```python
from build123d import *

# Parameters (mm, degrees)
F0_W     = 30
F0_H     = 100
F1_DEPTH = 10
F2_W     = 17
F2_H     = 10
F3_DEPTH = 200
F2_H_2   = 5
F4_DEPTH = 60
F5_R     = 1.25
F6_DEPTH = 25
F7_R     = 1.25
F8_DEPTH = 25


with BuildPart() as f1:
    # F0 (on Top) → F1 (new body, symmetric)
    with BuildSketch(Plane.XY):
        Rectangle(F0_W, F0_H)
    extrude(amount=F1_DEPTH, both=True)

    # F2 (on face) → F3 (cut)
    with BuildSketch(Plane.XZ.offset(50)):
        Rectangle(F2_W, F2_H)
    extrude(amount=-F3_DEPTH, mode=Mode.SUBTRACT)

    # F2 (on face) → F4 (cut)
    with BuildSketch(Plane.XZ.offset(50)):
        Polygon((8.5, 10), (8.5, 5), (8.5, -5), (10.5, -5), (10.5, 10), align=None)
        Polygon((-8.5, -5), (-8.5, 5), (-8.5, 10), (-10.5, 10), (-10.5, -5), align=None)
        with Locations((0, 7.5)):
            Rectangle(F2_W, F2_H_2)
    extrude(amount=-F4_DEPTH, mode=Mode.SUBTRACT)

    # F5 (on face) → F6 (cut)
    with BuildSketch(Plane.XY.offset(-5)):
        with Locations((0, -18.688429)):
            Circle(F5_R)
        with Locations((0, -40.465806)):
            Circle(F5_R)
    extrude(amount=-F6_DEPTH, mode=Mode.SUBTRACT)

    # F7 (on face) → F8 (cut)
    with BuildSketch(Plane.XY.offset(10)):
        with Locations((0, 30.281067)):
            Circle(F7_R)
    extrude(amount=-F8_DEPTH, mode=Mode.SUBTRACT)


solid = f1.part
```
Source: CAD feature listing. Evaluate the final solid. Frame: model axes, mm. A direction names the side the tool comes from. Round coordinates to 2 decimals unless told otherwise and drop trailing zeros. Loops run counter-clockwise (first coordinate to the right, second up) from the corner with the lowest first, then second, coordinate; pieces in that order, holes last.
1. Section query D-D on y = 36. Output: boundary loops of the cut face in (x, z).
2. Access query for faces 4 (the flat face through (0, -1, -5)), 5 (the flat face through (-10.5, -20, 3)), 6 (the flat face through (8.5, 30, 0)). Directions: +Z, -Z, +X, -X, +Y, -Y. A direction counts if a zero-diameter tool reaches every point of the face in a straight line with its end or side. Return the directions, or none.
3. Ray query, L1, parallel to Y at x = 0, z = -6.4; L2, parallel to X at y = 8, z = 5; L3, parallel to Z at x = -3, y = 28. Return the intervals inside material, ascending.
4. Section query C-C on x = -5.25. Output: boundary loops of the cut face in (y, z).
5. Section query B-B on z = -3. Output: boundary loops of the cut face in (x, y).
6. Mould query, pull axis Y, two halves, no side actions, for faces 1 (the flat face through (-15, -1, 0)), 2 (the cylindrical face through (-0.271, -41.686, -7.465)), 3 (the flat face through (0, 50, 7)). Classes: released by +Y, released by -Y, zero draft, split by the parting line, or undercut.
7. Section query A-A on x = 0. Output: boundary loops of the cut face in (y, z).
8. Contact query for flat-ended pins moving along their axis: pin 1 (12 mm diameter, centred on x = -1.5, z = 5.5, fed in from -Y); pin 2 (2 mm diameter, centred on x = 0, y = 30.28, fed in from +Z). Output: stop coordinate, or through.
Answers below:
1. outline: (-15, -10) - (15, -10) - (15, 10) - (-15, 10) - close; hole (-8.5, -5) - (8.5, -5) - (8.5, 5) - (-8.5, 5) - close
2. face 4: -Y
2. face 5: +Z, -Y
2. face 6: +Y, -Y
3. L1: y = -50 to -41.72, -39.22 to -19.94, -17.44 to 29.03, 31.53 to 50
3. L2: x = -15 to -10.5, 10.5 to 15
3. L3: z = -10 to -5, 5 to 10
4. outline: (-50, -10) - (50, -10) - (50, -5) - (-50, -5) - close; (10, 5) - (50, 5) - (50, 10) - (10, 10) - close
5. outline: (-15, -50) - (-10.5, -50) - (-10.5, 10) - (-8.5, 10) - (-8.5, 50) - (-15, 50) - close; (8.5, 10) - (10.5, 10) - (10.5, -50) - (15, -50) - (15, 50) - (8.5, 50) - close
6. face 1: zero draft
6. face 2: undercut
6. face 3: released by +Y
7. outline: (-50, -10) - (-41.72, -10) - (-41.72, -5) - (-50, -5) - close; (-39.22, -10) - (-19.94, -10) - (-19.94, -5) - (-39.22, -5) - close; (-17.44, -10) - (29.03, -10) - (29.03, -5) - (-17.44, -5) - close; (10, 5) - (29.03, 5) - (29.03, 10) - (10, 10) - close; (31.53, -10) - (50, -10) - (50, -5) - (31.53, -5) - close; (31.53, 5) - (50, 5) - (50, 10) - (31.53, 10) - close
8. pin 1: stops at y = 10
8. pin 2: passes through
